Input: part model. Units: mm. Frame: model coordinates. Coordinates: 2 decimals unless noted, no trailing zeros. Loops run counter-clockwise (first coordinate to the right, second up) from the corner with the lowest first, then second, coordinate; pieces in that order, holes last.
```python
from build123d import *

# Parameters (mm, degrees)
SKETCH1_R           = 57.5
SKETCH1_R_2         = 1.6
BOSS_EXTRUDE1_DEPTH = 10.6
FILLET1_R           = 5


with BuildPart() as part:
    # Sketch1 → Boss-Extrude1 (new body)
    with BuildSketch(Plane(origin=(0, 0, 0), x_dir=(1, 0, 0), z_dir=(0, 1, 0))):
        with Locations(Location((0, 0, 0), (0, 0, 270))):
            Circle(SKETCH1_R)
        with Locations(Location((-27, -46.765371804, 0), (0, 0, 270))):
            Circle(SKETCH1_R_2, mode=Mode.SUBTRACT)
        with Locations(Location((-46.765371804, -27, 0), (0, 0, 270))):
            Circle(SKETCH1_R_2, mode=Mode.SUBTRACT)
        with Locations(Location((-54, 0, 0), (0, 0, 270))):
            Circle(SKETCH1_R_2, mode=Mode.SUBTRACT)
        with Locations(Location((0, -54, 0), (0, 0, 270))):
            Circle(SKETCH1_R_2, mode=Mode.SUBTRACT)
        with Locations(Location((27, -46.765371804, 0), (0, 0, 270))):
            Circle(SKETCH1_R_2, mode=Mode.SUBTRACT)
        with BuildLine():
            ThreePointArc((43.742247125, 10.564838686), (44.135337618, 8.779064491), (44.455555556, 6.978795043))
            ThreePointArc((44.455555556, 6.978795043), (49.753361384, 5.138633627), (52, 0))
            ThreePointArc((52, 0), (49.753361384, -5.138633627), (44.455555556, -6.978795043))
            ThreePointArc((44.455555556, -6.978795043), (44.135337618, -8.779064491), (43.742247125, -10.564838686))
            ThreePointArc((43.742247125, -10.564838686), (47.23910353, -13.108193036), (48.574578963, -17.220754456))
            ThreePointArc((48.574578963, -17.220754456), (45.234108152, -23.187985482), (38.400908644, -23.459970489))
            ThreePointArc((38.400908644, -23.459970489), (37.416132554, -25.000660486), (36.369578094, -26.500071496))
            ThreePointArc((36.369578094, -26.500071496), (38.177808401, -28.89135937), (38.819805153, -31.819805153))
            ThreePointArc((38.819805153, -31.819805153), (34.244868492, -38.386316236), (26.500071496, -36.369578094))
            ThreePointArc((26.500071496, -36.369578094), (25.000660486, -37.416132554), (23.459970489, -38.400908644))
            ThreePointArc((23.459970489, -38.400908644), (24.027901885, -39.942787345), (24.220754456, -41.574578963))
            ThreePointArc((24.220754456, -41.574578963), (18.318158122, -48.488022764), (10.564838686, -43.742247125))
            ThreePointArc((10.564838686, -43.742247125), (8.779064491, -44.135337618), (6.978795043, -44.455555556))
            ThreePointArc((6.978795043, -44.455555556), (6.994696752, -44.727571384), (7, -45))
            ThreePointArc((7, -45), (-0.272428616, -51.994696752), (-6.978795043, -44.455555556))
            ThreePointArc((-6.978795043, -44.455555556), (-8.779064491, -44.135337618), (-10.564838686, -43.742247125))
            ThreePointArc((-10.564838686, -43.742247125), (-19.899538483, -48.041735691), (-23.459970489, -38.400908644))
            ThreePointArc((-23.459970489, -38.400908644), (-25.000660486, -37.416132554), (-26.500071496, -36.369578094))
            ThreePointArc((-26.500071496, -36.369578094), (-36.769552622, -36.769552622), (-36.369578094, -26.500071496))
            ThreePointArc((-36.369578094, -26.500071496), (-37.416132554, -25.000660486), (-38.400908644, -23.459970489))
            ThreePointArc((-38.400908644, -23.459970489), (-48.041735691, -19.899538483), (-43.742247125, -10.564838686))
            ThreePointArc((-43.742247125, -10.564838686), (-44.135337618, -8.779064491), (-44.455555556, -6.978795043))
            ThreePointArc((-44.455555556, -6.978795043), (-52, 0), (-44.455555556, 6.978795043))
            ThreePointArc((-44.455555556, 6.978795043), (-44.135337618, 8.779064491), (-43.742247125, 10.564838686))
            ThreePointArc((-43.742247125, 10.564838686), (-48.041735691, 19.899538483), (-38.400908644, 23.459970489))
            ThreePointArc((-38.400908644, 23.459970489), (-37.416132554, 25.000660486), (-36.369578094, 26.500071496))
            ThreePointArc((-36.369578094, 26.500071496), (-36.769552622, 36.769552622), (-26.500071496, 36.369578094))
            ThreePointArc((-26.500071496, 36.369578094), (-25.000660486, 37.416132554), (-23.459970489, 38.400908644))
            ThreePointArc((-23.459970489, 38.400908644), (-19.899538483, 48.041735691), (-10.564838686, 43.742247125))
            ThreePointArc((-10.564838686, 43.742247125), (-8.779064491, 44.135337618), (-6.978795043, 44.455555556))
            ThreePointArc((-6.978795043, 44.455555556), (-0.272428616, 51.994696752), (7, 45))
            ThreePointArc((7, 45), (6.994696752, 44.727571384), (6.978795043, 44.455555556))
            ThreePointArc((6.978795043, 44.455555556), (8.779064491, 44.135337618), (10.564838686, 43.742247125))
            ThreePointArc((10.564838686, 43.742247125), (18.318158122, 48.488022764), (24.220754456, 41.574578963))
            ThreePointArc((24.220754456, 41.574578963), (24.027901885, 39.942787345), (23.459970489, 38.400908644))
            ThreePointArc((23.459970489, 38.400908644), (25.000660486, 37.416132554), (26.500071496, 36.369578094))
            ThreePointArc((26.500071496, 36.369578094), (34.244868492, 38.386316236), (38.819805153, 31.819805153))
            ThreePointArc((38.819805153, 31.819805153), (38.177808401, 28.89135937), (36.369578094, 26.500071496))
            ThreePointArc((36.369578094, 26.500071496), (37.416132554, 25.000660486), (38.400908644, 23.459970489))
            ThreePointArc((38.400908644, 23.459970489), (45.234108152, 23.187985482), (48.574578963, 17.220754456))
            ThreePointArc((48.574578963, 17.220754456), (47.23910353, 13.108193036), (43.742247125, 10.564838686))
        make_face(mode=Mode.SUBTRACT)
        with Locations(Location((46.765371804, -27, 0), (0, 0, 270))):
            Circle(SKETCH1_R_2, mode=Mode.SUBTRACT)
        with Locations(Location((-46.765371804, 27, 0), (0, 0, 270))):
            Circle(SKETCH1_R_2, mode=Mode.SUBTRACT)
        with Locations(Location((-27, 46.765371804, 0), (0, 0, 270))):
            Circle(SKETCH1_R_2, mode=Mode.SUBTRACT)
        with Locations(Location((54, 0, 0), (0, 0, 270))):
            Circle(SKETCH1_R_2, mode=Mode.SUBTRACT)
        with Locations(Location((46.765371804, 27, 0), (0, 0, 270))):
            Circle(SKETCH1_R_2, mode=Mode.SUBTRACT)
        with Locations(Location((0, 54, 0), (0, 0, 270))):
            Circle(SKETCH1_R_2, mode=Mode.SUBTRACT)
        with Locations(Location((27, 46.765371804, 0), (0, 0, 270))):
            Circle(SKETCH1_R_2, mode=Mode.SUBTRACT)
    extrude(amount=BOSS_EXTRUDE1_DEPTH)

    # Fillet1
    # the kernel refuses this fillet: 5 mm, written as the material it takes off along each edge
    with BuildSketch(Plane(origin=(-23.459970489, -8.409987516, -38.400908644), x_dir=(-0.2723938397119589, 0, -0.9621858428011585), z_dir=(0, 1, 0)), Plane(origin=(-36.369578094, -8.409987516, -26.500071496), x_dir=(-0.6198716741882146, 0, -0.7847031971000881), z_dir=(0, 1, 0)), Plane(origin=(-43.742247125, -8.409987516, -10.564838686), x_dir=(-0.8729796654201095, 0, -0.48775660299271545), z_dir=(0, 1, 0)), Plane(origin=(-44.455555556, -8.409987516, 6.978795043), x_dir=(-0.9931844161721819, 0, -0.11655348760428477), z_dir=(0, 1, 0)), Plane(origin=(-26.500071496, -8.409987516, 36.369578094), x_dir=(-0.7847031971000193, 0, 0.6198716741883018), z_dir=(0, 1, 0)), Plane(origin=(-10.564838686, -8.409987516, 43.742247125), x_dir=(-0.4877566029925422, 0, 0.8729796654202064), z_dir=(0, 1, 0)), Plane(origin=(6.978795043, -8.409987516, 44.455555556), x_dir=(-0.11655348760405627, 0, 0.9931844161722087), z_dir=(0, 1, 0)), Plane(origin=(23.459970489, -8.409987516, 38.400908644), x_dir=(0.2723938397121838, 0, 0.9621858428010948), z_dir=(0, 1, 0)), Plane(origin=(36.369578094, -8.409987516, 26.500071496), x_dir=(0.6198716741885055, 0, 0.7847031970998585), z_dir=(0, 1, 0)), Plane(origin=(43.742247125, -8.409987516, 10.564838686), x_dir=(0.8729796654202305, 0, 0.48775660299249896), z_dir=(0, 1, 0)), Plane(origin=(44.455555556, -8.409987516, -6.978795043), x_dir=(0.993184416172219, 0, 0.11655348760396912), z_dir=(0, 1, 0)), Plane(origin=(38.400908644, -8.409987516, -23.459970489), x_dir=(0.9621858428010855, 0, -0.2723938397122163), z_dir=(0, 1, 0)), Plane(origin=(26.500071496, -8.409987516, -36.369578094), x_dir=(0.7847031970998928, 0, -0.6198716741884621), z_dir=(0, 1, 0)), Plane(origin=(10.564838686, -8.409987516, -43.742247125), x_dir=(0.4877566029926196, 0, -0.8729796654201631), z_dir=(0, 1, 0)), Plane(origin=(-6.978795043, -8.409987516, -44.455555556), x_dir=(0.11655348760419053, 0, -0.9931844161721929), z_dir=(0, 1, 0))) as fillet1_piece_1:
        with BuildLine():
            CenterArc((3.675513735, 4.905552558), FILLET1_R, 199.899092777, 58.946827573)
            ThreePointArc((-1.025953847, 3.20372925), (-0.483029435, 1.61145493), (0, 0))
            ThreePointArc((0, 0), (1.354136639, 0.132226419), (2.708273278, 0))
        make_face()
    extrude(amount=27.419975032, mode=Mode.SUBTRACT)
    with BuildSketch(Plane(origin=(-26.500071496, -8.409987516, -36.369578094), x_dir=(0.8296594592290296, 0, -0.5582698108547461), z_dir=(0, 1, 0)), Plane(origin=(-38.400908644, -8.409987516, -23.459970489), x_dir=(0.5528647859323804, 0, -0.8332709814195759), z_dir=(0, 1, 0)), Plane(origin=(-44.455555556, -8.409987516, -6.978795043), x_dir=(0.1919014607092957, 0, -0.9814141986835317), z_dir=(0, 1, 0)), Plane(origin=(-43.742247125, -8.409987516, 10.564838686), x_dir=(-0.19827712231571695, 0, -0.9801460007397867), z_dir=(0, 1, 0)), Plane(origin=(-36.369578094, -8.409987516, 26.500071496), x_dir=(-0.558269810854761, 0, -0.8296594592290196), z_dir=(0, 1, 0)), Plane(origin=(-23.459970489, -8.409987516, 38.400908644), x_dir=(-0.8332709814195962, 0, -0.5528647859323499), z_dir=(0, 1, 0)), Plane(origin=(-6.978795043, -8.409987516, 44.455555556), x_dir=(-0.9814141986835541, 0, -0.19190146070918135), z_dir=(0, 1, 0)), Plane(origin=(10.564838686, -8.409987516, 43.742247125), x_dir=(-0.9801460007397754, 0, 0.1982771223157732), z_dir=(0, 1, 0)), Plane(origin=(26.500071496, -8.409987516, 36.369578094), x_dir=(-0.8296594592289986, 0, 0.5582698108547921), z_dir=(0, 1, 0)), Plane(origin=(38.400908644, -8.409987516, 23.459970489), x_dir=(-0.552864785932314, 0, 0.83327098141962), z_dir=(0, 1, 0)), Plane(origin=(44.455555556, -8.409987516, 6.978795043), x_dir=(-0.19190146070922567, 0, 0.9814141986835454), z_dir=(0, 1, 0)), Plane(origin=(43.742247125, -8.409987516, -10.564838686), x_dir=(0.19827712231576203, 0, 0.9801460007397778), z_dir=(0, 1, 0)), Plane(origin=(23.459970489, -8.409987516, -38.400908644), x_dir=(0.8332709814195809, 0, 0.552864785932373), z_dir=(0, 1, 0)), Plane(origin=(6.978795043, -8.409987516, -44.455555556), x_dir=(0.9814141986835359, 0, 0.19190146070927452), z_dir=(0, 1, 0)), Plane(origin=(-10.564838686, -8.409987516, -43.742247125), x_dir=(0.9801460007397866, 0, -0.1982771223157175), z_dir=(0, 1, 0))) as fillet1_piece_2:
        with BuildLine():
            CenterArc((3.550883618, 4.996506044), FILLET1_R, 208.911087711, 58.946827573)
            ThreePointArc((-0.825971318, 2.579247086), (-0.287058705, 1.329950061), (0, 0))
            ThreePointArc((0, 0), (1.681997503, 0.031445605), (3.363995006, 0))
        make_face()
    extrude(amount=27.419975032, mode=Mode.SUBTRACT)
    with BuildSketch(Plane(origin=(36.369578094, -8.409987516, -26.500071496), x_dir=(0.6198716741884495, 0, -0.7847031970999027), z_dir=(0, 1, 0))) as fillet1_piece_3:
        with BuildLine():
            CenterArc((3.675513735, -4.905552558), FILLET1_R, 101.154079649, 58.946827573)
            ThreePointArc((-1.025953847, -3.20372925), (-0.483029435, -1.61145493), (0, 0))
            ThreePointArc((0, 0), (1.354136639, -0.132226419), (2.708273278, 0))
        make_face()
    extrude(amount=27.419975032, mode=Mode.SUBTRACT)


solid = part.part
```
Item 1: Section query A-A (x = 0). Output: boundary loops of the cut face in (y, z).
Result:
outline: (0, -57.5) - (10.6, -57.5) - (10.6, -55.6) - (0, -55.6) - close; (0, -52.4) - (10.6, -52.4) - (10.6, -52) - (0, -52) - close; (0, 52) - (10.6, 52) - (10.6, 52.4) - (0, 52.4) - close; (0, 55.6) - (10.6, 55.6) - (10.6, 57.5) - (0, 57.5) - close
Item 2: Line query: L1, parallel to X at y = 3.25, z = -27; L2, parallel to X at y = 6.25, z = -47.5; L3, parallel to X at y = 9.25, z = -39. Output: solid intervals per line, ascending.
Result:
L1: x = -50.77 to -48.37, -45.17 to -37.54, 37.54 to 45.17, 48.37 to 50.77
L2: x = -32.4 to -28.42, -25.58 to -20.95, -13.49 to -6.54, 6.54 to 13.49, 20.95 to 25.58, 28.42 to 32.4
L3: x = -42.25 to -24.44, 24.44 to 42.25
Item 3: Section query B-B (z = -5). Output: boundary loops of the cut face in (x, y), then the cut area to 3 significant figures.
Result:
outline: (-57.28, 0) - (-49.9, 0) - (-49.9, 10.6) - (-57.28, 10.6) - close; (49.9, 0) - (57.28, 0) - (57.28, 10.6) - (49.9, 10.6) - close
area: 157 mm2
Item 4: Contact query for flat-ended pins moving along their axis: P1, Ø1.9, axis at x = -46.77, z = -27, coming from the -Y side; P2, Ø1.5, axis at x = -35.5, y = 6, coming from the +Z side; P3, Ø1.5, axis at x = 9, y = 6.5, coming from the -Z side; P4, Ø1.5, axis at y = 6, z = -42.5, coming from the -X side. Output: stop coordinate, or through.
Result:
P1: passes through
P2: stops at z = 45.81
P3: stops at z = -56.91
P4: stops at x = -39.54
Item 5: Section query C-C (x = -17). Output: boundary loops of the cut face in (y, z).
Result:
outline: (0, -54.93) - (10.6, -54.93) - (10.6, -48.57) - (0, -48.57) - close; (0, 48.57) - (10.6, 48.57) - (10.6, 54.93) - (0, 54.93) - close
Item 6: Section query D-D (z = -27). Output: boundary loops of the cut face in (x, y), then the cut area to 3 significant figures.
Result:
outline: (-50.77, 0) - (-48.37, 0) - (-48.37, 10.6) - (-50.77, 10.6) - close; (-45.17, 0) - (-37.54, 0) - (-37.54, 10.6) - (-45.17, 10.6) - close; (37.54, 0) - (45.17, 0) - (45.17, 10.6) - (37.54, 10.6) - close; (48.37, 0) - (50.77, 0) - (50.77, 10.6) - (48.37, 10.6) - close
area: 213 mm2
